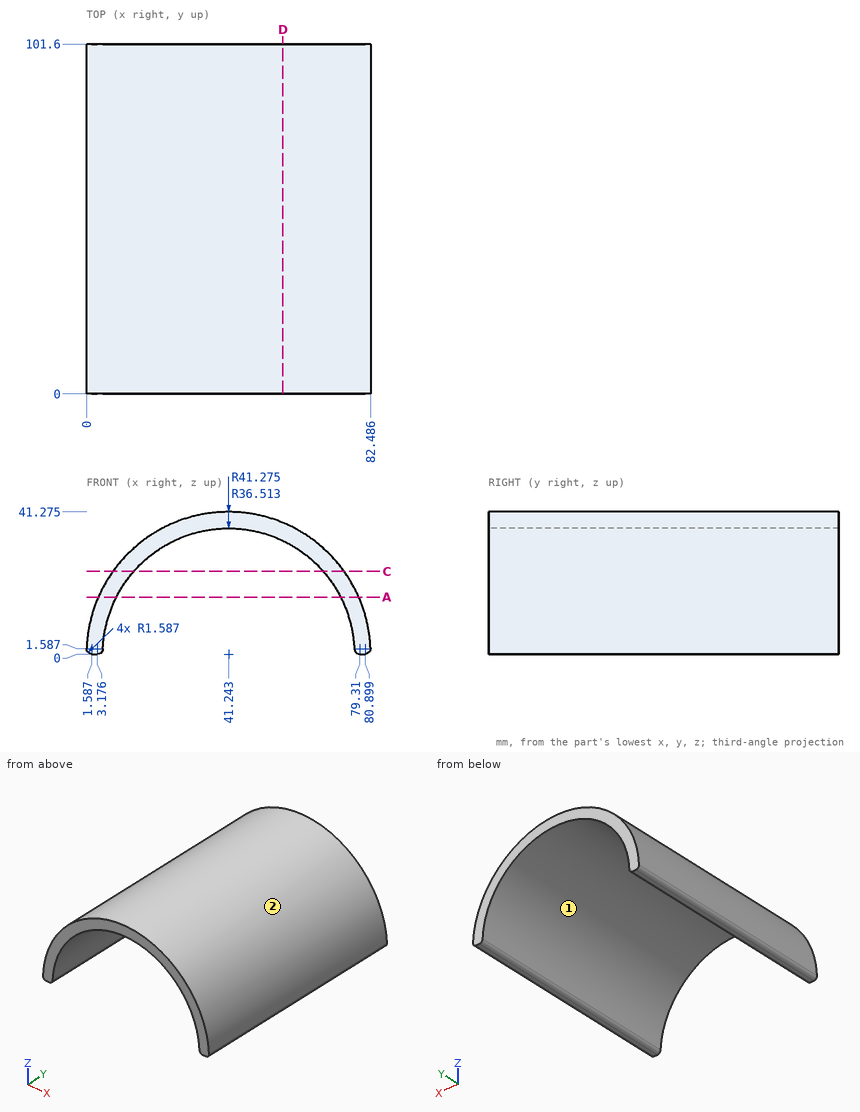
Can you work these out from the drawing? Everything is in mm from the part's minimum corner. Round coordinates to 2 decimals unless told otherwise and drop trailing zeros. Write each loop counter-clockwise with the first axis right and the second up, starting at its lowest first coordinate (ties: lowest second). Pieces come first, ordered by that corner, then holes.
1. Will these pins go through, and if not, where does the flat tip stop? pin 1 Ø2 at (x, y) = (28.5, 80) entering from +Z; pin 2 Ø4 at (y, z) = (51, 29) entering from +X; pin 3 Ø4 at (x, z) = (74, 4) entering from -Y; pin 4 Ø12 at (y, z) = (63, 22.5) entering from +X.
2. I need wall thicknesses on L1, parallel to X at y = 76.5, z = 7 (1 decimal); L2, parallel to X at y = 49, z = 28 (1 decimal); L3, parallel to Z at x = 61.5, y = 8. Which ranges of each line are inside material? Lowest first, please.
3. Suppose I cut it at D-D (x = 57). List the corners of the cut face in (y, z) for me.
4. Suppose I cut it at C-C (z = 24). List the corners of the cut face in (x, y) for me, and give its area (3 significant figures).
5. If we mould it in two halves opening along X, with no side actions, what happens to the marked faces 1 and 2? For each: released by +X, released by -X, zero draft, split by the parting line, or undercut.
6. Suppose I cut it at A-A (z = 16.5). List the corners of the cut face in (x, y) for me (1 decimal), and give its area (3 significant figures).
Answer sheet:
1. pin 1: stops at z = 39.57
1. pin 2: stops at x = 72.46
1. pin 3: passes through
1. pin 4: stops at x = 79.08
2. L1: x = 0.6 to 5.4, 77.1 to 81.9
2. L2: x = 10.9 to 17.8, 64.7 to 71.6
2. L3: z = 30.38 to 35.96
3. outline: (0, 32.94) - (101.6, 32.94) - (101.6, 38.15) - (0, 38.15) - close
4. outline: (7.66, 0) - (13.73, 0) - (13.73, 101.6) - (7.66, 101.6) - close; (68.76, 0) - (74.82, 0) - (74.82, 101.6) - (68.76, 101.6) - close
4. area: 1,230 mm2
5. face 1: undercut
5. face 2: split by the parting line
6. outline: (3.4, 0) - (8.7, 0) - (8.7, 101.6) - (3.4, 101.6) - close; (73.8, 0) - (79.1, 0) - (79.1, 101.6) - (73.8, 101.6) - close
6. area: 1,070 mm2
